from build123d import *

# Parameters (mm, degrees)
BOSS_EXTRUDE1_DEPTH    = 23
BOSS_EXTRUDE2_DEPTH    = 11
BOSS_EXTRUDE3_START    = 5
SKETCH1_4_R            = 5.000000000000004
BOSS_EXTRUDE3_DEPTH    = 6
BOSS_EXTRUDE4_START    = -11
SKETCH1_5_R            = 5.000000000000004
BOSS_EXTRUDE4_DEPTH    = 6
BOSS_EXTRUDE5_DEPTH    = 7.5
FILLET1_RADIUS         = 7.5
FILLET1_LENGTH         = 6
FILLET2_RADIUS         = 7.5
FILLET2_LENGTH         = 6
F_10_0MM_DOWEL_HOLE1_D = 10


with BuildPart() as part:
    # Sketch1 → Boss-Extrude1 (new, symmetric)
    with BuildSketch(Plane(origin=(0, 0, 0), x_dir=(0, 0, -1), z_dir=(1, 0, 0))):
        with BuildLine():
            ThreePointArc((18, 0), (14.696938456699069, 10.392304845413266), (5.999999999999998, 16.97056274847714))
            ThreePointArc((5.999999999999998, 16.97056274847714), (-6.763446053329629, 16.68100109357049), (-16.1245154965971, 8.000000000000002))
            ThreePointArc((-16.1245154965971, 8.000000000000002), (-17.269106839051002, 5.077198930654761), (-17.888543819998286, 2.0000000000002958))
            Line((-17.888543819998254, 1.9999999999999998), (-12.845232578665128, 2.0000000000000004))
            ThreePointArc((-12.845232578665128, 2.0000000000000018), (1.0029896503337725, 12.96125039343517), (13, 0))
            ThreePointArc((13, -3.18e-15), (1.0029896503337692, -12.96125039343517), (-12.84523257866513, -1.9999999999999987))
            Line((-12.845232578665128, -2.0000000000000004), (-17.888543819998254, -1.9999999999999998))
            ThreePointArc((-17.888543819998286, -2.0000000000002918), (-17.269106839051005, -5.077198930654757), (-16.124515496597102, -7.999999999999997))
            ThreePointArc((-16.124515496597102, -7.999999999999997), (-6.763446053329637, -16.681001093570487), (5.999999999999995, -16.970562748477143))
            ThreePointArc((5.999999999999995, -16.970562748477143), (14.69693845669907, -10.39230484541326), (18, -4.41e-15))
        make_face()
    extrude(amount=BOSS_EXTRUDE1_DEPTH, both=True)

    # Sketch1<3> → Boss-Extrude2 (add, symmetric)
    with BuildSketch(Plane(origin=(0, 0, 0), x_dir=(0, 0, -1), z_dir=(1, 0, 0))):
        with BuildLine():
            Line((21.000000000000004, 11.667261889578032), (6, 16.97056274847714))
            ThreePointArc((5.999999999999998, 16.97056274847714), (14.696938456699069, 10.392304845413266), (18, 0))
            ThreePointArc((18, -4.41e-15), (14.69693845669907, -10.39230484541326), (5.999999999999995, -16.970562748477143))
            Line((6, -16.97056274847714), (21.000000000000004, -11.667261889578032))
            Line((21.000000000000004, -11.66726188957803), (21.000000000000004, 11.66726188957803))
        make_face()
    extrude(amount=BOSS_EXTRUDE2_DEPTH, both=True)

    # Sketch1<4> → Boss-Extrude3 (add)
    with BuildSketch(Plane(origin=(0, 0, 0), x_dir=(0, 0, -1), z_dir=(1, 0, 0)).offset(BOSS_EXTRUDE3_START)):
        with BuildLine():
            Line((35.333333333333336, 6.599663291074442), (21.000000000000004, 11.667261889578032))
            Line((21.000000000000004, 11.66726188957803), (21.000000000000004, -11.66726188957803))
            Line((21.000000000000004, -11.667261889578032), (35.333333333333336, -6.599663291074442))
            ThreePointArc((35.333333333333336, -6.59966329107444), (40, -2.2e-16), (35.333333333333336, 6.5996632910744415))
        make_face()
        with Locations((33, 0)):
            Circle(SKETCH1_4_R, mode=Mode.SUBTRACT)
    extrude(amount=BOSS_EXTRUDE3_DEPTH)

    # Sketch1<5> → Boss-Extrude4 (add)
    with BuildSketch(Plane(origin=(0, 0, 0), x_dir=(0, 0, -1), z_dir=(1, 0, 0)).offset(BOSS_EXTRUDE4_START)):
        with BuildLine():
            Line((35.333333333333336, 6.599663291074442), (21.000000000000004, 11.667261889578032))
            Line((21.000000000000004, 11.66726188957803), (21.000000000000004, -11.66726188957803))
            Line((21.000000000000004, -11.667261889578032), (35.333333333333336, -6.599663291074442))
            ThreePointArc((35.333333333333336, -6.59966329107444), (40, -2.2e-16), (35.333333333333336, 6.5996632910744415))
        make_face()
        with Locations((33, 0)):
            Circle(SKETCH1_5_R, mode=Mode.SUBTRACT)
    extrude(amount=BOSS_EXTRUDE4_DEPTH)

    # Sketch1<7> → Boss-Extrude5 (add, symmetric)
    with BuildSketch(Plane(origin=(0, 0, 0), x_dir=(0, 0, -1), z_dir=(1, 0, 0))):
        with BuildLine():
            Line((-35, -7.999999999999998), (-16.1245154965971, -7.9999999999999964))
            ThreePointArc((-16.124515496597102, -7.999999999999997), (-17.269106839051005, -5.077198930654757), (-17.888543819998286, -2.0000000000002918))
            Line((-17.888543819998254, -1.9999999999999998), (-35, -1.9999999999999973))
            Line((-35, -1.9999999999999973), (-35, -7.999999999999998))
        make_face()
        with BuildLine():
            ThreePointArc((-17.888543819998286, 2.0000000000002958), (-17.269106839051002, 5.077198930654761), (-16.1245154965971, 8.000000000000002))
            Line((-16.1245154965971, 7.9999999999999964), (-35, 7.999999999999998))
            Line((-35, 7.999999999999998), (-35, 1.9999999999999973))
            Line((-35, 1.9999999999999973), (-17.888543819998254, 1.9999999999999998))
        make_face()
    extrude(amount=BOSS_EXTRUDE5_DEPTH, both=True)

    # Fillet1: full round fillet: the end face becomes a half cylinder, R = half its width
    fillet1_face = Plane((0, -5, 35), x_dir=(0, -1, 0), z_dir=(0, 0, 1))  # on the end face: x along it, z out of the body
    fillet1_slab = fillet1_face.offset(-FILLET1_RADIUS / 2) * Box(FILLET1_LENGTH, 2 * FILLET1_RADIUS, FILLET1_RADIUS, mode=Mode.PRIVATE)  # the body's end, R deep
    fillet1_round = Plane((0, -5, 27.5), x_dir=(0, 0, 1), z_dir=(0, -1, 0)) * Cylinder(FILLET1_RADIUS, FILLET1_LENGTH, mode=Mode.PRIVATE)  # its axis R under the face
    add(fillet1_slab - fillet1_round, mode=Mode.SUBTRACT)

    # Fillet2: full round fillet: the end face becomes a half cylinder, R = half its width
    fillet2_face = Plane((0, 5, 35), x_dir=(0, -1, 0), z_dir=(0, 0, 1))  # on the end face: x along it, z out of the body
    fillet2_slab = fillet2_face.offset(-FILLET2_RADIUS / 2) * Box(FILLET2_LENGTH, 2 * FILLET2_RADIUS, FILLET2_RADIUS, mode=Mode.PRIVATE)  # the body's end, R deep
    fillet2_round = Plane((0, 5, 27.5), x_dir=(0, 0, 1), z_dir=(0, -1, 0)) * Cylinder(FILLET2_RADIUS, FILLET2_LENGTH, mode=Mode.PRIVATE)  # its axis R under the face
    add(fillet2_slab - fillet2_round, mode=Mode.SUBTRACT)

    # Ø10.0mm Dowel Hole1 (through all)
    with Locations(Plane(origin=(0, -8, 27.5), x_dir=(0, 0, -1), z_dir=(0, -1, 0))):
        with Locations((0, 0)):
            Hole(F_10_0MM_DOWEL_HOLE1_D / 2)


solid = part.part
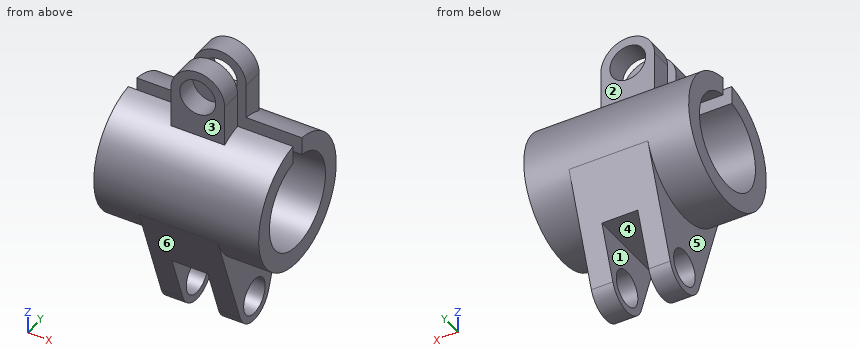
Can you work these out from the model? Positions are in its coordinate system, mm. Face numbers are marked on the shaded views. A direction names the side the tool comes from. Coordinates: 2 decimals unless noted, no trailing zeros. Loops run counter-clockwise (first coordinate to the right, second up) from the corner with the lowest first, then second, coordinate; pieces in that order, holes last. Notation, with made-up numbers: M -0.5,15.5 L 47.5,15.5 A11 cw 47.5,24.5 Z; hole C -33,56 d7. An arc over 180 degrees is marked long. Return JSON: item names as keys, results as strings. Group by question number.
Item 1: Imagine slicing it at B-B (x = 0). Please give me the cut outline in (y, z).
Item 2: Imagine slicing it at C-C (y = -3.5). Give the number of separate pieces and of enclosed holes in the cut face, and give its area (3 significant figures).
Item 3: Imagine slicing it at A-A (z = 19.5). Please give me the cut outline in (x, y).
Item 4: If I drill on L1, parallel to Y at x = 5, z = 0; L2, parallel to X at y = -4.5, z = -25; L3, parallel to Y at x = -5, z = 30.5, over which ranges is the centre line in solid material (lowest first)? Write a range as from..to.
Item 5: I'm going to push flat-ended pins straight in: pin 1 Ø15 at (y, z) = (3.5, -30.5) entering from -X; pin 2 Ø12 at (x, z) = (-2, 29.5) entering from +Y; pin 3 Ø4 at (x, z) = (-6.5, 21.5) entering from -Y. Where does each tip first touch, or does it pass through?
Item 6: On a 3-axis mill with a long thin cutter (end or side, diameter ignored), from which of +Z, -Z, +X, -X, +Y, -Y can I reach the whole of each face in a straight line? I mean the marked faces 1, 2 and 3. Say none if no direction works.
Item 7: Thinking about a two-plate mould opening in X: for the marked faces 4, 5 and 6, which applies, released by +X, released by -X, zero draft, split by the parting line, or undercut?
Item 8: Imagine slicing it at D-D (x = -10). Please give me the cut outline in (y, z).
Verdict:
{
 "1": {"outline": "M -16.97,-6 L -11.67,-21 L 11.67,-21 L 16.97,-6 A18 ccw 8,16.12 L 8,22.5 L 2,22.5 L 2,12.85 A13 cw long -2,12.85 L -2,22.5 L -8,22.5 L -8,16.12 A18 ccw Z; M -8,32.5 L -2,32.5 L -2,35 L -8,35 Z; M 2,32.5 L 8,32.5 L 8,35 L 2,35 Z"},
 "2": {"separate pieces": "4", "enclosed holes": "1", "area": "835 mm^2"},
 "3": {"outline": "M -7.5,-8 L 7.5,-8 L 7.5,-2 L -7.5,-2 Z; M -7.5,2 L 7.5,2 L 7.5,8 L -7.5,8 Z"},
 "4": {"L1": "y = -18..-13, 13..18", "L2": "x = -11..-5, 5..11", "L3": "y = -8..-2, 2..8"},
 "5": {"pin 1": "stops at x = -11", "pin 2": "stops at y = 8", "pin 3": "stops at y = -8"},
 "6": {"face 1": "-Z, +Y, -Y", "face 2": "+Z, +X, -X, +Y", "face 3": "+Z, +X, -X, -Y"},
 "7": {"face 4": "undercut", "face 5": "released by -X", "face 6": "zero draft"},
 "8": {"outline": "M -16.97,-6 L -6.6,-35.33 A7 ccw 6.6,-35.33 L 16.97,-6 A18 ccw 2,17.89 L 2,12.85 A13 cw long -2,12.85 L -2,17.89 A18 ccw Z; hole C 0,-33 d10"}
}
